Geometry: final body of the model. Coordinates: model frame, mm. Face numbers are marked on the shaded views. A direction names the side the tool comes from. Give positions to 0.01 mm unless a question says otherwise; leave off trailing zeros. Order: outer loops, then holes, each group sorted by start corner. A loop starts at its lowest first (then second) coordinate and runs counter-clockwise, first axis right, second up. Notation, with made-up numbers: (89.25, 7) -> (124.25, 7) arc R19 ccw to (124.25, 28) -> close; hole circle Ø4 at (-36, -4). An arc over 180 degrees is marked (long way). Answer in a Markdown table with one row per item. Add a question column.
Q1. Contact query for flat-ended pins moving along their axis: P1, Ø3, axis at x = 6, z = -0.5, coming from the -Y side; P2, Ø0.7, axis at y = -1, z = 0.5, coming from the -X side; P3, Ø2, axis at x = 6.5, y = 1.5, coming from the +Z side; P4, Ø2, axis at x = 4, y = -1.5, coming from the -Z side. Output: stop coordinate, or through.
Q2. Cut plane B-B on x = -1. Return the cut outline in (y, z).
Q3. Line query: line 1 along Y through (x, z) = (0.05, 0); line 2 along X through (y, z) = (1, -2). Output: solid intervals per line, ascending. Write a range as from..to.
Q4. Pull-direction query (Z, two-part tool) for the marked faces 1, 2 and 3; classes: +Z half, -Z half, draft (parallel to the pull), parting line (faces both ways), or undercut.
Q5. Set-up query: the marked faces 4 and 5. Return all of +Z, -Z, +X, -X, +Y, -Y with unobstructed straight access to the full face (end or side cutting, diameter ignored); none if empty.
Q6. Cut plane A-A on x = 6.25. Return the cut outline in (y, z).
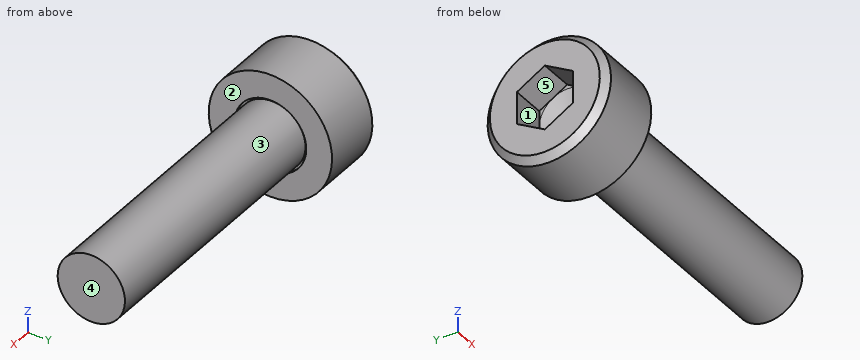
from build123d import *

# Parameters (mm, degrees)
SKETCH_1_W          = 3
SKETCH_1_H          = 2.75
SKETCH_2_R          = 1.5
EXTRUDE_1_DEPTH     = 100
CUT_EXTRUDE_1_DEPTH = 1.5
CHAMFER_1_SIZE      = 0.3
CUT_EXTRUDE_START   = -0.1
SKETCH_5_R          = 1.6
SKETCH_5_R_2        = 1.5
CUT_EXTRUDE_2_DEPTH = 0.1


with BuildPart() as part:
    # ｽｹｯﾁ1 → 回転1 (revolve)
    with BuildSketch(Plane.XY, mode=Mode.PRIVATE) as revolve_1_sk:
        with Locations((-1.5, 1.375)):
            Rectangle(SKETCH_1_W, SKETCH_1_H)
    revolve(revolve_1_sk.sketch.rotate(Axis((-3, 0, 0), (1, 0, 0)), 270), axis=Axis((-3, 0, 0), (1, 0, 0)))

    # ｽｹｯﾁ2 → ﾎﾞｽ - 押し出し1 (add)
    with BuildSketch(Plane(origin=(0, 0, 0), x_dir=(0, 0, -1), z_dir=(1, 0, 0))):
        Circle(SKETCH_2_R)
    extrude(amount=EXTRUDE_1_DEPTH)

    # ｽｹｯﾁ3 → ｶｯﾄ - 押し出し1 (cut)
    with BuildSketch(Plane.ZY.offset(3)):
        Polygon((-0.72, -1.247076581), (0.72, -1.247076581), (1.44, 0), (0.72, 1.247076581), (-0.72, 1.247076581), (-1.44, 0), align=None)
    extrude(amount=-CUT_EXTRUDE_1_DEPTH, mode=Mode.SUBTRACT)

    # ｽｹｯﾁ4 → ｶｯﾄ - 回転1 (revolve, cut)
    with BuildSketch(Plane.XY, mode=Mode.PRIVATE) as cut_revolve_1_sk:
        Polygon((-1.5, 1.247076581), (-1.5, 0), (-1.165063509, 0), align=None)
    revolve(cut_revolve_1_sk.sketch.rotate(Axis((-1.500025, 0, 0), (1, 0, 0)), 90), axis=Axis((-1.500025, 0, 0), (1, 0, 0)), mode=Mode.SUBTRACT)

    # 面取り1
    chamfer_1_edges = [part.edges().sort_by_distance(p)[0] for p in [
        (100, 0, 1.5),
        (-3, 0, 2.75),
    ]]
    chamfer(chamfer_1_edges, length=CHAMFER_1_SIZE)

    # ｽｹｯﾁ5 → ｶｯﾄ - 押し出し2 (cut)
    with BuildSketch(Plane(origin=(0, 0, 0), x_dir=(0, 0, -1), z_dir=(1, 0, 0)).offset(CUT_EXTRUDE_START)):
        Circle(SKETCH_5_R)
        Circle(SKETCH_5_R_2, mode=Mode.SUBTRACT)
    extrude(amount=CUT_EXTRUDE_2_DEPTH, mode=Mode.SUBTRACT)

    # Surface Cut 14
    split(bisect_by=Plane(origin=(12, 0, 0), x_dir=(0, 0, -1), z_dir=(1, 0, 0)), keep=Keep.BOTTOM)


solid = part.part
Completed:
| question | item | result |
|---|---|---|
| 1 | P1 | stops at y = -1.5 |
| 1 | P2 | stops at x = -3 |
| 1 | P3 | stops at z = 1.41 |
| 1 | P4 | stops at z = -1.41 |
| 2 | outline | circle Ø5.5 at (0, 0) |
| 3 | line 1 | y = -1.5..1.5 |
| 3 | line 2 | x = -3..0 |
| 4 | face 1 | undercut |
| 4 | face 2 | draft |
| 4 | face 3 | parting line |
| 5 | face 4 | +Z, -Z, +X, +Y, -Y |
| 5 | face 5 | -X |
| 6 | outline | circle Ø3 at (0, 0) |
